Source: CAD feature listing. Evaluate the final solid. Frame: model axes, mm. Round coordinates to 2 decimals unless told otherwise and drop trailing zeros. Loops run counter-clockwise (first coordinate to the right, second up) from the corner with the lowest first, then second, coordinate; pieces in that order, holes last. Notation, with made-up numbers: M -15,30 L 24,30 A24 cw 24,66 Z; hole C 75.5,18.5 d11. An arc over 180 degrees is marked long. One line per item, written item: value.
from build123d import *

# Parameters (mm, degrees)
SKETCH1_W           = 214
SKETCH1_H           = 186
BOSS_EXTRUDE1_DEPTH = 3


with BuildPart() as part:
    # Sketch1 → Boss-Extrude1 (new body)
    with BuildSketch(Plane(origin=(0, 0, 0), x_dir=(1, 0, 0), z_dir=(0, 1, 0))):
        Rectangle(SKETCH1_W, SKETCH1_H)
        Polygon((-82, 83), (82, 83), (97, 68), (97, -68), (82, -83), (-82, -83), (-97, -68), (-97, 68), align=None, mode=Mode.SUBTRACT)
    extrude(amount=BOSS_EXTRUDE1_DEPTH)


solid = part.part
1. Ray query, line 1 (Z direction, x = -30.5, y = 2.45); line 2 (X direction, y = 2.95, z = -43); line 3 (Z direction, x = -93.5, y = 1.7). Return the intervals inside material, ascending. Write a range as [from, to].
Report:
line 1: z = [-93, -83], [83, 93]
line 2: x = [-107, -97], [97, 107]
line 3: z = [-93, -71.5], [71.5, 93]
2. Section query B-B (y = 0.6). Return the cut outline in (x, z).
Report:
outline: M -107,-93 L 107,-93 L 107,93 L -107,93 Z; hole M -97,-68 L -82,-83 L 82,-83 L 97,-68 L 97,68 L 82,83 L -82,83 L -97,68 Z
3. Section query A-A (x = 92). Return the cut outline in (y, z).
Report:
outline: M 0,-93 L 3,-93 L 3,-73 L 0,-73 Z; M 0,73 L 3,73 L 3,93 L 0,93 Z
4. Section query C-C (z = 43). Return the cut outline in (x, y).
Report:
outline: M -107,0 L -97,0 L -97,3 L -107,3 Z; M 97,0 L 107,0 L 107,3 L 97,3 Z
